```python
from build123d import *

# Parameters (mm, degrees)
SKETCH_1_R            = 2.5
EXTRUDE_19_DEPTH      = 2.1
EXTRUDE_START         = 1
SKETCH_1_24_R         = 9
SKETCH_1_24_R_2       = 2.5
EXTRUDE_20_DEPTH      = 1
EXTRUDE_21_DEPTH      = 1
EXTRUDE_21_DEPTH_BACK = 2.1
SKETCH_1_25_R         = 10
SKETCH_1_25_R_2       = 9
FILLET_1_R            = 1
FILLET_2_R            = 0.5
FILLET_3_R            = 0.5
FILLET_4_R            = 1


with BuildPart() as part:
    # 草图1 → 凸台-拉伸19 (new body)
    with BuildSketch(Plane.XY):
        Circle(SKETCH_1_R)
        Polygon((0.57030636, 0.535854496), (0.57030636, 2.2), (-0.57030636, 2.2), (-0.57030636, 0.535854496), (-2.2, 0.535854496), (-2.2, -0.535854496), (-0.57030636, -0.535854496), (-0.57030636, -2.2), (0.57030636, -2.2), (0.57030636, -0.535854496), (2.2, -0.535854496), (2.2, 0.535854496), align=None, mode=Mode.SUBTRACT)
    extrude(amount=-EXTRUDE_19_DEPTH)

    # 草图1<24> → 凸台-拉伸20 (add)
    # profile 1 of 4: a face of its own
    with BuildSketch(Plane.XY.offset(EXTRUDE_START)):
        Circle(SKETCH_1_24_R)
        Circle(SKETCH_1_24_R_2, mode=Mode.SUBTRACT)
    # profile 2 of 4: a face of its own
    with BuildSketch(Plane.XY.offset(EXTRUDE_START)):
        Circle(SKETCH_1_24_R_2)
        Polygon((0.57030636, 0.535854496), (0.57030636, 2.2), (-0.57030636, 2.2), (-0.57030636, 0.535854496), (-2.2, 0.535854496), (-2.2, -0.535854496), (-0.57030636, -0.535854496), (-0.57030636, -2.2), (0.57030636, -2.2), (0.57030636, -0.535854496), (2.2, -0.535854496), (2.2, 0.535854496), align=None, mode=Mode.SUBTRACT)
    # profile 3 of 4: a face of its own
    with BuildSketch(Plane.XY.offset(EXTRUDE_START)):
        Polygon((0.57030636, 0.535854496), (2.2, 0.535854496), (2.2, -0.535854496), (0.57030636, -0.535854496), (0.57030636, -2.2), (-0.57030636, -2.2), (-0.57030636, -0.535854496), (-2.2, -0.535854496), (-2.2, 0.535854496), (-0.57030636, 0.535854496), (-0.57030636, 2.2), (0.57030636, 2.2), align=None)
        Polygon((0.37030636, -0.335854496), (2, -0.335854496), (2, 0.335854496), (0.37030636, 0.335854496), (0.37030636, 2), (-0.37030636, 2), (-0.37030636, 0.335854496), (-2, 0.335854496), (-2, -0.335854496), (-0.37030636, -0.335854496), (-0.37030636, -2), (0.37030636, -2), align=None, mode=Mode.SUBTRACT)
    # profile 4 of 4: a face of its own
    with BuildSketch(Plane.XY.offset(EXTRUDE_START)):
        Polygon((0.37030636, -2), (0.37030636, -0.335854496), (2, -0.335854496), (2, 0.335854496), (0.37030636, 0.335854496), (0.37030636, 2), (-0.37030636, 2), (-0.37030636, 0.335854496), (-2, 0.335854496), (-2, -0.335854496), (-0.37030636, -0.335854496), (-0.37030636, -2), align=None)
    extrude(amount=-EXTRUDE_20_DEPTH)

    # 草图1<25> → 凸台-拉伸21 (add, two sides: drawn at the far end of the back side and taken through both)
    with BuildSketch(Plane.XY.offset(-EXTRUDE_21_DEPTH_BACK)):
        Circle(SKETCH_1_25_R)
        Circle(SKETCH_1_25_R_2, mode=Mode.SUBTRACT)
    extrude(amount=EXTRUDE_21_DEPTH + EXTRUDE_21_DEPTH_BACK)

    # 圆角1
    fillet_1_edges = [part.edges().sort_by_distance(p)[0] for p in [
        (-10, 0, 1),
    ]]
    fillet(fillet_1_edges, radius=FILLET_1_R - 0.0001)  # a hair under: the kernel refuses the full size

    # 圆角2
    fillet_2_edges = [part.edges().sort_by_distance(p)[0] for p in [
        (-10, 0, -2.1),
    ]]
    fillet(fillet_2_edges, radius=FILLET_2_R)

    # 圆角3
    fillet_3_edges = [part.edges().sort_by_distance(p)[0] for p in [
        (-9, 0, -2.1),
    ]]
    fillet(fillet_3_edges, radius=FILLET_3_R - 0.0001)  # a hair under: the kernel refuses the full size

    # 圆角4
    fillet_4_edges = [part.edges().sort_by_distance(p)[0] for p in [
        (-9, 0, 0),
    ]]
    fillet(fillet_4_edges, radius=FILLET_4_R)


solid = part.part
```
Verification items for the finished model (mm, model axes). A direction names the side the tool comes from. Coordinates: 2 decimals unless noted, no trailing zeros. Order: outer loops, then holes, each group sorted by start corner. A loop starts at its lowest first (then second) coordinate and runs counter-clockwise, first axis right, second up. Notation, with made-up numbers: (70, 88.5) -> (108, 88.5) arc R19 cw to (108, 116.5) -> close; hole circle Ø8 at (3.25, 12). An arc over 180 degrees is marked (long way). Answer as CSV lines item,"result". Start each with the question number.
1) Release check for a two-part mould opening along X. For faces 1 (the face through (-1, 0.536, -1)), 2 (the face through (-2.17, -9.76, -0.81)), 3 (the face through (0, 0, 1)) record: released by +X, released by -X, zero draft, split by the parting line, or undercut.
2) Material ranges on L1, parallel to Y at x = 0, z = -1.05; L2, parallel to X at y = -1.75, z = -1.9; L3, parallel to Z at x = 0.5, y = -1.75, recorded low to high. Write a range as [from, to].
3) Cross-section at A-A, the plane z = -1.3. Record the boundary of the cut face in (x, y).
4) Gauge pin test, flat ends, axial feed: pin 1 Ø1 at (x, z) = (4, -1) entering from -Y; pin 2 Ø0.8 at (x, z) = (-1, -1.5) entering from +Y; pin 3 Ø1.3 at (x, z) = (1.5, -1.5) entering from -Y. Record the tip position at first contact, or that the pin passes through.
5) Cross-section at D-D, the plane z = -0.3. Record the boundary of the cut face in (x, y), then the cut area to 3 significant figures.
6) Set-up check for faces 4 (the face through (-1, 1, -2.1)), 5 (the face through (-1, -0.536, -1)): record each of +Z, -Z, +X, -X, +Y, -Y from which the full face is reachable in a straight line by a thin tool's end or side.
Conclusion:
1,face 1,"undercut"
1,face 2,"split by the parting line"
1,face 3,"zero draft"
2,L1,"y = [-10, -9], [-2.5, -2.2], [2.2, 2.5], [9, 10]"
2,L2,"x = [-9.74, -8.93], [-1.79, -0.57], [0.57, 1.79], [8.93, 9.74]"
2,L3,"z = [0, 1]"
3,outline,"circle Ø20 at (0, 0); circle Ø5 at (0, 0); hole circle Ø18 at (0, 0); hole (-2.2, -0.54) -> (-0.57, -0.54) -> (-0.57, -2.2) -> (0.57, -2.2) -> (0.57, -0.54) -> (2.2, -0.54) -> (2.2, 0.54) -> (0.57, 0.54) -> (0.57, 2.2) -> (-0.57, 2.2) -> (-0.57, 0.54) -> (-2.2, 0.54) -> close"
4,pin 1,"stops at y = -9.37"
4,pin 2,"stops at y = 9.98"
4,pin 3,"stops at y = -9.96"
5,outline,"circle Ø20 at (0, 0); circle Ø5 at (0, 0); hole circle Ø17.43 at (0, 0); hole (-2.2, -0.54) -> (-0.57, -0.54) -> (-0.57, -2.2) -> (0.57, -2.2) -> (0.57, -0.54) -> (2.2, -0.54) -> (2.2, 0.54) -> (0.57, 0.54) -> (0.57, 2.2) -> (-0.57, 2.2) -> (-0.57, 0.54) -> (-2.2, 0.54) -> close"
5,area,"86.7 mm²"
6,face 4,"-Z, +X, -X, +Y, -Y"
6,face 5,"-Z"
